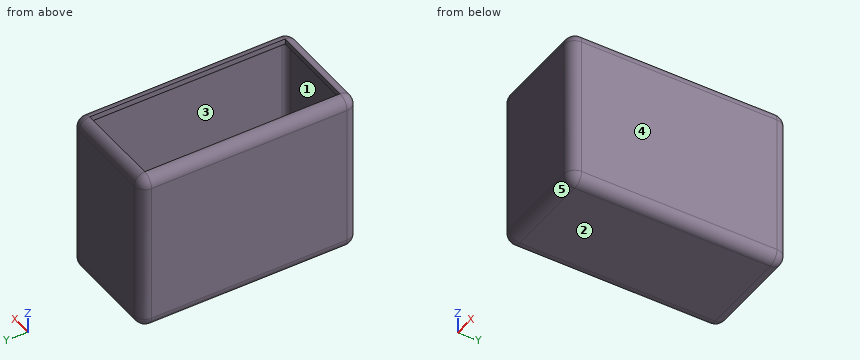
from build123d import *

# Parameters (mm, degrees)
F0_W     = 50.8
F0_H     = 101.6
F1_DEPTH = 76.2
F2_R     = 5.08
F3_T     = -2.54


# Not quite as in the source:
# - a shell that OpenCascade refuses in one call is made with other operations: the cavity is built on its own and cut out


with BuildPart() as f1:
    # F0 (on Top) → F1 (new body)
    with BuildSketch(Plane.XY):
        Rectangle(F0_W, F0_H)
    extrude(amount=F1_DEPTH)

    # F2
    f2_edges = [f1.edges().sort_by_distance(p)[0] for p in [
        (-25.4, 0, 76.2),
        (0, 50.8, 76.2),
        (-25.4, 50.8, 38.1),
        (-25.4, -50.8, 38.1),
        (0, -50.8, 76.2),
        (25.4, 0, 76.2),
        (25.4, -50.8, 38.1),
        (25.4, 50.8, 38.1),
        (0, 50.8, 0),
        (25.4, 0, 0),
        (-25.4, 0, 0),
        (0, -50.8, 0),
    ]]
    fillet(f2_edges, radius=F2_R)

    # F3: a shell. OpenCascade refuses it in one call, so the cavity is built on its own and cut out:
    # the body offset inwards by the wall thickness, plus a prism from it out through each open face.
    f3_core = offset(f1.part, amount=F3_T, mode=Mode.PRIVATE)
    f3_exits = [f3_core.faces().sort_by_distance(p)[0] for p in [
        (0, 0, 73.66),
    ]]
    add(f3_core, mode=Mode.SUBTRACT)
    extrude(f3_exits, amount=-F3_T, mode=Mode.SUBTRACT)


solid = f1.part
Part model, mm, in its own coordinate system. Face numbers are marked on the shaded views. A direction names the side the tool comes from. Round coordinates to 2 decimals unless told otherwise and drop trailing zeros. Order: outer loops, then holes, each group sorted by start corner. A loop starts at its lowest first (then second) coordinate and runs counter-clockwise, first axis right, second up. Notation, with made-up numbers: (-17.5, -26) -> (-3.5, -26) arc R13 ccw to (-3.5, -14) -> close; hole circle Ø5 at (23, -34.5). An arc over 180 degrees is marked (long way). Put each result on its own line as item: value.
Q1. Pin check, flat tips, straight feed: pin 1 Ø12 at (x, y) = (-6, 21) entering from +Z; pin 2 Ø2 at (y, z) = (4, 75) entering from +X; pin 3 Ø3 at (x, z) = (7, 74.5) entering from -Y. Stop position of each tip, or through.
From the geometry:
pin 1: stops at z = 2.54
pin 2: stops at x = 24.5
pin 3: stops at y = -50.44
Q2. Band-saw the part on C-C (y = -1.5). Give the cut face in (x, z).
From the geometry:
outline: (-25.4, 5.08) arc R5.08 ccw to (-20.32, 0) -> (20.32, 0) arc R5.08 ccw to (25.4, 5.08) -> (25.4, 71.12) arc R5.08 ccw to (20.32, 76.2) -> (20.32, 73.66) arc R2.54 cw to (22.86, 71.12) -> (22.86, 5.08) arc R2.54 cw to (20.32, 2.54) -> (-20.32, 2.54) arc R2.54 cw to (-22.86, 5.08) -> (-22.86, 71.12) arc R2.54 cw to (-20.32, 73.66) -> (-20.32, 76.2) arc R5.08 ccw to (-25.4, 71.12) -> close
Q3. Band-saw the part on A-A (z = 47). Give the cut face in (x, y), and give its area (3 significant figures).
From the geometry:
outline: (-25.4, -45.72) arc R5.08 ccw to (-20.32, -50.8) -> (20.32, -50.8) arc R5.08 ccw to (25.4, -45.72) -> (25.4, 45.72) arc R5.08 ccw to (20.32, 50.8) -> (-20.32, 50.8) arc R5.08 ccw to (-25.4, 45.72) -> close; hole (-22.86, -45.72) arc R2.54 ccw to (-20.32, -48.26) -> (20.32, -48.26) arc R2.54 ccw to (22.86, -45.72) -> (22.86, 45.72) arc R2.54 ccw to (20.32, 48.26) -> (-20.32, 48.26) arc R2.54 ccw to (-22.86, 45.72) -> close
area: 732 mm2
Q4. Band-saw the part on B-B (x = -2). Give the cut face in (y, z), and give its area (3 significant figures).
From the geometry:
outline: (-50.8, 5.08) arc R5.08 ccw to (-45.72, 0) -> (45.72, 0) arc R5.08 ccw to (50.8, 5.08) -> (50.8, 71.12) arc R5.08 ccw to (45.72, 76.2) -> (45.72, 73.66) arc R2.54 cw to (48.26, 71.12) -> (48.26, 5.08) arc R2.54 cw to (45.72, 2.54) -> (-45.72, 2.54) arc R2.54 cw to (-48.26, 5.08) -> (-48.26, 71.12) arc R2.54 cw to (-45.72, 73.66) -> (-45.72, 76.2) arc R5.08 ccw to (-50.8, 71.12) -> close
area: 629 mm2
Q5. Tool access for the marked faces 1 and 2: list every direction of +Z, -Z, +X, -X, +Y, -Y with a clear straight run to the whole face (end or side of a thin tool).
From the geometry:
face 1: none
face 2: -Z, +X, -X, +Y, -Y
Q6. Pull direction X, two halves, no side cores. Call the marked faces 3, 4 and 5: pulls with the +X half, pulls with the -X half, needs draft (parallel to the pull), parting line crosses it, or undercut.
From the geometry:
face 3: undercut
face 4: pulls with the +X half
face 5: needs draft
Q7. Wall check: line 1 (Y direction, x = -17, z = 16.5); line 2 (X direction, y = -39.5, z = 9.5); line 3 (Z direction, x = 12, y = 8.5). Give the ranges that are in metal, low to high. Write a range as [from, to].
From the geometry:
line 1: y = [-50.8, -48.26], [48.26, 50.8]
line 2: x = [-25.4, -22.86], [22.86, 25.4]
line 3: z = [0, 2.54]
